Geometry: final body of the model. Coordinates: model frame, mm. Give positions to 0.01 mm unless a question says otherwise; leave off trailing zeros. Loops run counter-clockwise (first coordinate to the right, second up) from the corner with the lowest first, then second, coordinate; pieces in that order, holes last. Notation, with made-up numbers: M 36,30.5 L 42,30.5 A12 cw 42,34.5 Z; hole C -13,83 d5. An arc over 180 degrees is marked long. Put each result on its own line as item: value.
```python
from build123d import *

# Parameters (mm, degrees)
F0_R          = 25
F0_W          = 8.1
F0_H          = 8.1
F1_DEPTH      = 8
F2_R          = 1.65
F3_DEPTH      = 10
F3_DEPTH_BACK = 7
F4_SIZE2      = 7
F4_SIZE       = 1
F5_ANGLE      = 90


with BuildPart() as f1:
    # F0 (on Front) → F1 (new body)
    with BuildSketch(Plane.XZ):
        Circle(F0_R)
        Rectangle(F0_W, F0_H, mode=Mode.SUBTRACT)
    extrude(amount=F1_DEPTH)

    # F2 (on face) → F3 (cut, two sides)
    with BuildSketch(Plane.XZ.offset(8)) as f3_sk:
        with Locations((0, 22.5)):
            Circle(F2_R)
        with Locations((-4.678013, 22.008321)):
            Circle(F2_R)
        with Locations((-9.151574, 20.554773)):
            Circle(F2_R)
        with Locations((-13.225168, 18.202882)):
            Circle(F2_R)
        with Locations((-16.720759, 15.055439)):
            Circle(F2_R)
        with Locations((-19.485572, 11.25)):
            Circle(F2_R)
        with Locations((-21.398772, 6.952882)):
            Circle(F2_R)
        with Locations((-22.376743, 2.35189)):
            Circle(F2_R)
        with Locations((-22.376743, -2.35189)):
            Circle(F2_R)
        with Locations((-21.398772, -6.952882)):
            Circle(F2_R)
        with Locations((-19.485572, -11.25)):
            Circle(F2_R)
        with Locations((-16.720759, -15.055439)):
            Circle(F2_R)
        with Locations((-13.225168, -18.202882)):
            Circle(F2_R)
        with Locations((-9.151574, -20.554773)):
            Circle(F2_R)
        with Locations((-4.678013, -22.008321)):
            Circle(F2_R)
        with Locations((0, -22.5)):
            Circle(F2_R)
        with Locations((4.678013, -22.008321)):
            Circle(F2_R)
        with Locations((9.151574, -20.554773)):
            Circle(F2_R)
        with Locations((13.225168, -18.202882)):
            Circle(F2_R)
        with Locations((16.720759, -15.055439)):
            Circle(F2_R)
        with Locations((19.485572, -11.25)):
            Circle(F2_R)
        with Locations((21.398772, -6.952882)):
            Circle(F2_R)
        with Locations((22.376743, -2.35189)):
            Circle(F2_R)
        with Locations((22.376743, 2.35189)):
            Circle(F2_R)
        with Locations((21.398772, 6.952882)):
            Circle(F2_R)
        with Locations((19.485572, 11.25)):
            Circle(F2_R)
        with Locations((16.720759, 15.055439)):
            Circle(F2_R)
        with Locations((13.225168, 18.202882)):
            Circle(F2_R)
        with Locations((9.151574, 20.554773)):
            Circle(F2_R)
        with Locations((4.678013, 22.008321)):
            Circle(F2_R)
    extrude(amount=F3_DEPTH, mode=Mode.SUBTRACT)
    extrude(f3_sk.sketch, amount=-F3_DEPTH_BACK, mode=Mode.SUBTRACT)

    # F4
    f4_edges = [f1.edges().sort_by_distance(p)[0] for p in [
        (-25, 0, 0),
    ]]
    chamfer(f4_edges, length=F4_SIZE, length2=F4_SIZE2)


with BuildPart() as f1_1:
    # F5: moved
    add(f1.part.rotate(Axis((0, -8, 4.05), (-1, 0, 0)), F5_ANGLE))


solid = f1_1.part
```
Item 1: Section B-B on y = -12.05. Output: boundary loops of the cut face in (x, z).
Output values:
outline: M -25,-2.95 L -18,-3.95 L -4.05,-3.95 L -4.05,4.05 L -25,4.05 Z; M 4.05,-3.95 L 18,-3.95 L 25,-2.95 L 25,4.05 L 4.05,4.05 Z
Item 2: Section C-C on z = -0.25. Count the separate pieces of the cut face and the enclosed holes in it, then the cut area to 3 significant figures.
Output values:
separate pieces: 1
enclosed holes: 31
area: 1,640 mm²
Item 3: Section A-A on x = 0. Output: boundary loops of the cut face in (y, z).
Output values:
outline: M -37.05,-2.95 L -30.05,-3.95 L -16.1,-3.95 L -16.1,4.05 L -32.9,4.05 L -32.9,-2.95 L -36.2,-2.95 L -36.2,4.05 L -37.05,4.05 Z; M -8,-3.95 L 5.95,-3.95 L 12.95,-2.95 L 12.95,4.05 L 12.1,4.05 L 12.1,-2.95 L 8.8,-2.95 L 8.8,4.05 L -8,4.05 Z
Item 4: Pin query (flat end, axial travel): pin 1 Ø4 at (y, z) = (1.5, -2.5) entering from +X; pin 2 Ø4 at (x, y) = (22.38, -9.7) entering from -Z; pin 3 Ø2 at (y, z) = (-10.5, 2.5) entering from -X. Return the tip coordinate at first contact, or that it passes through.
Output values:
pin 1: x = 22.17
pin 2: z = -3.59
pin 3: x = -24.99
Item 5: Line query: probe 1 along Y at (x, z) = (21.5, 3); probe 2 along Y at (x, z) = (-19.5, -2.25); probe 3 along Y at (x, z) = (-5, 2.5). Output: solid intervals per line, ascending. Write a range as [from, to].
Output values:
probe 1: [-24.81, -20.65], [-17.36, -15.8], [-13, -11.1], [-8.3, -6.74], [-3.45, 0.71]
probe 2: [-27.69, -24.95], [-21.65, -2.45], [0.85, 3.59]
probe 3: [-36.54, -35.68], [-32.44, 8.34], [11.58, 12.44]
Item 6: Mould query, pull axis Y, two halves, no side actions, for faces 1 (the flat face through (-4.05, -12, 0)), 2 (the cylindrical face through (-7.63, 7.87, 0.6)). Classes: pulls with the +Y half, pulls with the -Y half, needs draft (parallel to the pull), parting line crosses it, or undercut.
Output values:
face 1: undercut
face 2: undercut
